```python
from build123d import *

# Parameters (mm, degrees)
BOSS_EXTRUDE1_DEPTH = 10
CIRPATTERN1_COUNT   = 18
CUT_EXTRUDE1_DEPTH  = 18.271256217


with BuildPart() as part:
    # Sketch1 → Boss-Extrude1 (new body)
    with BuildSketch(Plane(origin=(0, 0, 0), x_dir=(1, 0, 0), z_dir=(0, 1, 0))):
        with BuildLine():
            Line((7.969557585, 0.697245942), (8.965752283, 0.784401685))
            ThreePointArc((8.965752283, 0.784401685), (9.497437113, 0.667153604), (9.990482216, 0.436193874))
            ThreePointArc((9.990482216, 0.436193874), (10, 0), (9.990482216, -0.436193874))
            ThreePointArc((9.990482216, -0.436193874), (9.497437113, -0.667153604), (8.965752283, -0.784401685))
            Line((8.965752283, -0.784401685), (7.969557585, -0.697245942))
            ThreePointArc((7.969557585, -0.697245942), (7.931558891, -1.044209538), (7.878462024, -1.389185421))
            Line((7.878462024, -1.389185421), (0, 0))
            Line((0, 0), (7.878462024, 1.389185421))
            ThreePointArc((7.878462024, 1.389185421), (7.931558891, 1.044209538), (7.969557585, 0.697245942))
        make_face()
    boss_extrude1 = extrude(amount=BOSS_EXTRUDE1_DEPTH)

    # CirPattern1: Boss-Extrude1 ×18 about axis
    cirpattern1_axis = Axis((0, 0, 0), (0, 1, 0))
    for i in range(1, CIRPATTERN1_COUNT):
        add(boss_extrude1.rotate(cirpattern1_axis, i * 360 / CIRPATTERN1_COUNT))

    # Sketch6 → Cut-Extrude1 (cut, through all)
    with BuildSketch(Plane.XZ):
        with BuildLine():
            Line((-2.14, 1.93), (2.14, 1.93))
            ThreePointArc((2.14, 1.93), (2.868460939, 0), (2.14, -1.93))
            Line((2.14, -1.93), (-2.14, -1.93))
            ThreePointArc((-2.14, -1.93), (-2.868460939, 0), (-2.14, 1.93))
        make_face()
    extrude(amount=-CUT_EXTRUDE1_DEPTH, mode=Mode.SUBTRACT)


solid = part.part
```
Read the model definition and answer for the solid it produces. Units are mm, in the model's axes. A direction names the side the tool comes from. Coordinates: 2 decimals unless noted, no trailing zeros. Loops run counter-clockwise (first coordinate to the right, second up) from the corner with the lowest first, then second, coordinate; pieces in that order, holes last.
(1) The mould has two halves that part along X. Classify faces 1 (the face through (8.47, 4.93, 0.74)), 2 (the face through (-9.395, 4.93, 3.426)), 3 (the face through (8.204, 4.93, 2.198)): released by +X, released by -X, zero draft, split by the parting line, or undercut.
Solution:
face 1: undercut
face 2: released by -X
face 3: released by +X
(2) The part is cut by section A-A (x = -4.25). Determine the outline of the cut face in (y, z), and give its area (4 significant figures).
Solution:
outline: (0, -8.63) - (10, -8.63) - (10, 8.63) - (0, 8.63) - close
area: 172.5 mm2
(3) The part is cut by section B-B (z = -7). Determine the outline of the cut face in (x, y), and give its area (3 significant figures).
Solution:
outline: (-4.9, 0) - (4.9, 0) - (4.9, 10) - (-4.9, 10) - close
area: 98.0 mm2
(4) A tool of negligible diameter and unlimited length cuts with its end or side. For faces 4 (the face through (5.325, 4.93, 7.884)), 5 (the face through (-0.989, 4.93, 9.462)), 6 (the face through (-9.15, 4.93, -2.62)), 7 (the face through (0, 5, 1.93)), 8 (the face through (-4.177, 4.93, -8.564)), from which of +Z, -Z, +X, -X, +Y, -Y can it reach the whole face along a straight path? Write none if from no direction.
Solution:
face 4: +X, +Y, -Y
face 5: +Z, +Y, -Y
face 6: -X, +Y, -Y
face 7: +Y, -Y
face 8: -Z, +Y, -Y
(5) Flat-ended cylindrical pins translate along their axes: pin 1 Ø2 at (x, y) = (0.5, 4) entering from +Z; pin 2 Ø2 at (y, z) = (7, 3) entering from -X; pin 3 Ø1.3 at (x, y) = (0.5, 3.5) entering from +Z; pin 4 Ø4 at (x, y) = (-3.5, 4) entering from -Z. Find the tip coordinate at first contact, or state that the pin passes through.
Solution:
pin 1: stops at z = 9.91
pin 2: stops at x = -9.54
pin 3: stops at z = 9.72
pin 4: stops at z = -9.89
(6) Consider line 1 along Z through (x, y) = (0.25, 8.5); line 2 along Z through (x, y) = (5, 7) (3 decimals); line 3 along Z through (x, y) = (-1.5, 5.5). Determine where each line is inside the solid, lowest interval first.
Solution:
line 1: z = -8 to -1.93, 1.93 to 8
line 2: z = -8.66 to -7.141, -6.245 to 6.245, 7.141 to 8.66
line 3: z = -9.89 to -1.93, 1.93 to 9.89
